Input: dimensioned drawing with shaded views. Units: mm. Origin: part minimum x, y, z. A direction names the side the tool comes from. Round coordinates to 2 decimals unless told otherwise and drop trailing zeros. Loops run counter-clockwise (first coordinate to the right, second up) from the corner with the lowest first, then second, coordinate; pieces in that order, holes last. Notation, with made-up numbers: (45.25, 23.5) - (59.25, 23.5) arc R22 ccw to (59.25, 51.5) - close; hole circle Ø3 at (-37, -2.75). An arc over 180 degrees is marked (long way). One line per question, with ' | ' between items.
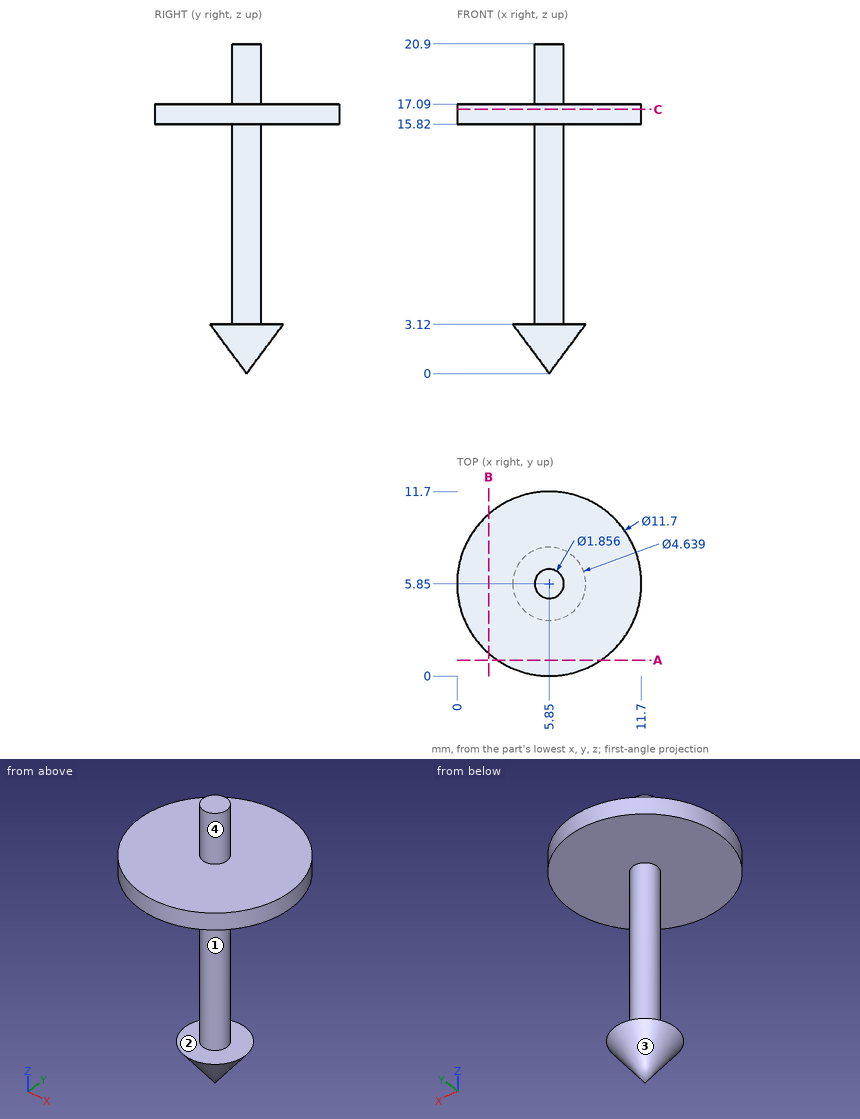
1. Access query for the marked faces 3 and 4. Directions: +Z, -Z, +X, -X, +Y, -Y. A direction counts if a zero-diameter tool reaches every point of the face in a straight line with its end or side. Return the directions, or none.
Worked out:
face 3: -Z | face 4: +Z
2. Contact query for flat-ended pins moving along their axis: P1, Ø1.5, axis at y = 5, z = 2, coming from the -X side; P2, Ø3, axis at x = 5.5, z = 13, coming from the -Y side; P3, Ø1.5, axis at x = 6, z = 2.5, coming from the -Y side. Output: stop coordinate, or through.
Worked out:
P1: stops at x = 3.93 | P2: stops at y = 4.92 | P3: stops at y = 3.53
3. Mould query, pull axis Y, two halves, no side actions, for the marked faces 1 and 2. Classes: released by +Y, released by -Y, zero draft, split by the parting line, or undercut.
Worked out:
face 1: split by the parting line | face 2: zero draft
4. Section query C-C, the plane z = 16.75. Return loops of the section in (x, y).
Worked out:
outline: circle Ø11.7 at (5.85, 5.85)
5. Section query B-B, the plane x = 2. Return loops of the section in (y, z) (1 decimal), plus the area to 3 significant figures.
Worked out:
outline: (1.4, 15.8) - (10.3, 15.8) - (10.3, 17.1) - (1.4, 17.1) - close | area: 11.2 mm2
6. Material intervals for probe 1 along Z at (x, y) = (7.25, 6.25); probe 2 along Z at (x, y) = (3, 1.75); probe 3 along Z at (x, y) = (5, 7.75), sorted ascending.
Worked out:
probe 1: z = 1.96 to 3.12, 15.82 to 17.09 | probe 2: z = 15.82 to 17.09 | probe 3: z = 2.8 to 3.12, 15.82 to 17.09
7. Section query A-A, the plane y = 1. Return loops of the section in (x, z).
Worked out:
outline: (2.58, 15.82) - (9.12, 15.82) - (9.12, 17.09) - (2.58, 17.09) - close
